Geometry check sheet. Reference: the model listing, model coordinates, mm. Coordinates: 2 decimals unless noted, no trailing zeros. Loops run counter-clockwise (first coordinate to the right, second up) from the corner with the lowest first, then second, coordinate; pieces in that order, holes last.
from build123d import *

# Parameters (mm, degrees)
BOSS_EXTRUDE1_DEPTH = 9.128125
SKETCH2_R           = 6.35
CUT_EXTRUDE1_DEPTH  = 1071.879363264


with BuildPart() as part:
    # Sketch1 → Boss-Extrude1 (new, symmetric)
    with BuildSketch(Plane.XY):
        with BuildLine():
            Line((0, 0), (406.4, 0))
            Line((406.4, 0), (406.4, 38.1))
            ThreePointArc((406.4, 38.1), (207.539140749, 196.40002074), (111.667415652, 431.8))
            Line((111.667415652, 431.8), (38.1, 990.6))
            Line((38.1, 990.6), (0, 990.6))
            Line((0, 990.6), (0, 0))
        make_face()
    extrude(amount=BOSS_EXTRUDE1_DEPTH, both=True)

    # Sketch2 → Cut-Extrude1 (cut, through all)
    with BuildSketch(Plane.XY.offset(9.128125)):
        with Locations((18.25625, 972.34375)):
            Circle(SKETCH2_R)
        with Locations((18.25625, 18.25625)):
            Circle(SKETCH2_R)
        with Locations((388.14375, 18.25625)):
            Circle(SKETCH2_R)
        with Locations((18.25625, 43.65625)):
            Circle(SKETCH2_R)
        with Locations((18.25625, 939.8)):
            Circle(SKETCH2_R)
        with Locations((18.25625, 914.4)):
            Circle(SKETCH2_R)
    extrude(amount=-CUT_EXTRUDE1_DEPTH, mode=Mode.SUBTRACT)


solid = part.part
(1) Sectioned sample at B-B on x = 184. Record the cut outline in (y, z), and give its area (3 significant figures).
Findings:
outline: (0, -9.13) - (230.72, -9.13) - (230.72, 9.13) - (0, 9.13) - close
area: 4,210 mm2
(2) Gauge pin test, flat ends, axial feed: pin 1 Ø8 at (x, z) = (113.5, -3) entering from -Y; pin 2 Ø4 at (x, z) = (363, -0.5) entering from +Y; pin 3 Ø10 at (x, y) = (388.14, 18.26) entering from +Z; pin 4 Ø8 at (y, z) = (363.5, 1) entering from +X. Record the tip position at first contact, or that the pin passes through.
Findings:
pin 1: stops at y = 0
pin 2: stops at y = 61
pin 3: passes through
pin 4: stops at x = 126.66
(3) Sectioned sample at C-C on y = 808. Record the cut outline in (x, z).
Findings:
outline: (0, -9.13) - (62.14, -9.13) - (62.14, 9.13) - (0, 9.13) - close
(4) Scan lines: L1, parallel to X at y = 939.8, z = -2.5; L2, parallel to Y at x = 210, z = 0; L3, parallel to Y at x = 294, z = 8. Record each from-to range of solid material in increasing order.
Findings:
L1: x = 0 to 11.91, 24.61 to 44.79
L2: y = 0 to 193.14
L3: y = 0 to 106.7
(5) Sectioned sample at A-A on z = -1.5. Record the cut outline in (x, y).
Findings:
outline: (0, 0) - (406.4, 0) - (406.4, 38.1) arc R502.17 cw to (111.67, 431.8) - (38.1, 990.6) - (0, 990.6) - close; hole circle Ø12.7 at (18.26, 18.26); hole circle Ø12.7 at (18.26, 43.66); hole circle Ø12.7 at (18.26, 914.4); hole circle Ø12.7 at (18.26, 939.8); hole circle Ø12.7 at (18.26, 972.34); hole circle Ø12.7 at (388.14, 18.26)
